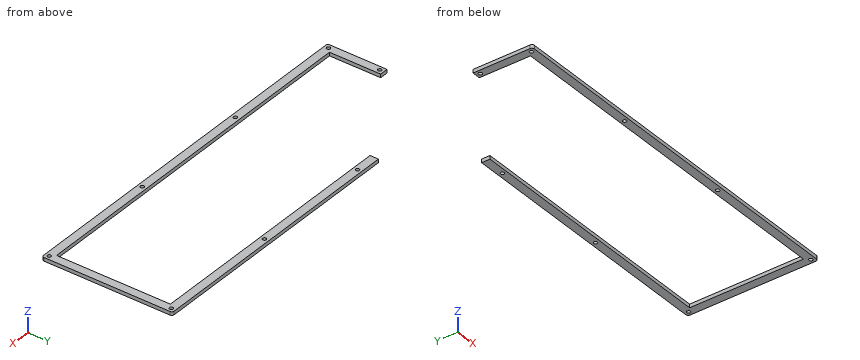
```python
from build123d import *

# Parameters (mm, degrees)
SKETCH_R  = 1.55
PAD_DEPTH = 3


with BuildPart() as part:
    # Sketch → Pad (new body)
    with BuildSketch(Plane.XY):
        with BuildLine():
            Line((71.8975, 17.4775), (301.2275, 17.4775))
            ThreePointArc((303.2275, 15.4775), (302.641714, 16.891714), (301.2275, 17.4775))
            Line((303.2275, 15.4775), (303.2275, -91.6775))
            ThreePointArc((301.2275, -93.6775), (302.641714, -93.091714), (303.2275, -91.6775))
            Line((301.2275, -93.6775), (-15.4775, -93.6775))
            ThreePointArc((-17.4775, -91.6775), (-16.891714, -93.091714), (-15.4775, -93.6775))
            Line((-17.4775, -91.6775), (-17.4775, -43.006))
            Line((-17.4775, -43.006), (-10.3335, -43.006))
            Line((-10.3335, -43.006), (-10.3335, -86.5335))
            Line((-10.3335, -86.5335), (296.0835, -86.5335))
            Line((296.0835, 10.3335), (296.0835, -86.5335))
            Line((71.8975, 10.3335), (296.0835, 10.3335))
            Line((71.8975, 17.4775), (71.8975, 10.3335))
        make_face()
        with Locations((-13.9055, -90.1055)):
            Circle(SKETCH_R, mode=Mode.SUBTRACT)
        with Locations((195.135167, -90.1055)):
            Circle(SKETCH_R, mode=Mode.SUBTRACT)
        with Locations((299.6555, -90.1055)):
            Circle(SKETCH_R, mode=Mode.SUBTRACT)
        with Locations((90.614833, -90.1055)):
            Circle(SKETCH_R, mode=Mode.SUBTRACT)
        with Locations((90.614833, 13.9055)):
            Circle(SKETCH_R, mode=Mode.SUBTRACT)
        with Locations((195.135167, 13.9055)):
            Circle(SKETCH_R, mode=Mode.SUBTRACT)
        with Locations((299.6555, 13.9055)):
            Circle(SKETCH_R, mode=Mode.SUBTRACT)
        with Locations((-13.9055, -46.578)):
            Circle(SKETCH_R, mode=Mode.SUBTRACT)
    extrude(amount=PAD_DEPTH)


solid = part.part
```
Geometry check sheet. Reference: the model listing, model coordinates, mm. Coordinates: 2 decimals unless noted, no trailing zeros. Loops run counter-clockwise (first coordinate to the right, second up) from the corner with the lowest first, then second, coordinate; pieces in that order, holes last. Notation, with made-up numbers: (81.25, -6) - (139.25, -6) arc R34 ccw to (139.25, 29) - close; hole circle Ø2 at (-36.75, 56). An arc over 180 degrees is marked (long way). One line per item, written item: value. Start each with the question number.
(1) Depth check by flat-ended pin: P1, Ø1.5, axis at y = -36.5, z = 1, coming from the -X side; P2, Ø0.9, axis at x = -15, z = 2, coming from the +Y side; P3, Ø3.5, axis at x = 195.14, y = -90.11, coming from the +Z side. Enter the tip coordinate at first touch or a pass-through.
(2) Cross-section at C-C on z = 0.65. Count the separate pieces of the cut face and the enclosed holes in it, plus the area to 3 significant figures.
(3) Material ranges on line 1 (Y direction, x = 214, z = 0.75); line 2 (X direction, y = 12.5, z = 1.3); line 3 (X direction, y = -48.5, z = 0.35), recorded low to high. Write a range as [from, to].
(4) Cross-section at B-B on x = 131.5. Enter the section's corners in (y, z), plus the area to 3 significant figures.
(5) Cross-section at A-A on y = -73. Enter the section's corners in (x, z).
(6) Cross-section at D-D on x = 8. Enter the section's corners in (y, z), plus the area to 3 significant figures.
Results below:
1. P1: stops at x = 296.08
1. P2: stops at y = -43.01
1. P3: stops at z = 3
2. separate pieces: 1
2. enclosed holes: 8
2. area: 4,880 mm2
3. line 1: y = [-93.68, -86.53], [10.33, 17.48]
3. line 2: x = [71.9, 89.96], [91.27, 194.48], [195.79, 299], [300.31, 303.23]
3. line 3: x = [-17.48, -10.33], [296.08, 303.23]
4. outline: (-93.68, 0) - (-86.53, 0) - (-86.53, 3) - (-93.68, 3) - close; (10.33, 0) - (17.48, 0) - (17.48, 3) - (10.33, 3) - close
4. area: 42.9 mm2
5. outline: (-17.48, 0) - (-10.33, 0) - (-10.33, 3) - (-17.48, 3) - close; (296.08, 0) - (303.23, 0) - (303.23, 3) - (296.08, 3) - close
6. outline: (-93.68, 0) - (-86.53, 0) - (-86.53, 3) - (-93.68, 3) - close
6. area: 21.4 mm2
